CAD build for the part. Positions are in the model's coordinates, mm. Face numbers are marked on the shaded views. A direction names the side the tool comes from. Give positions to 0.01 mm unless a question says otherwise; leave off trailing zeros. Write each loop counter-clockwise with the first axis right and the second up, starting at its lowest first coordinate (ties: lowest second). Pieces come first, ordered by that corner, then holes. Notation, with made-up numbers: (-5.75, 15) - (0.25, 15) arc R5 cw to (0.25, 22) - close; hole circle Ø10 at (70.25, 30.5). An arc over 180 degrees is marked (long way). Answer as a JSON object with one key per item and string values.
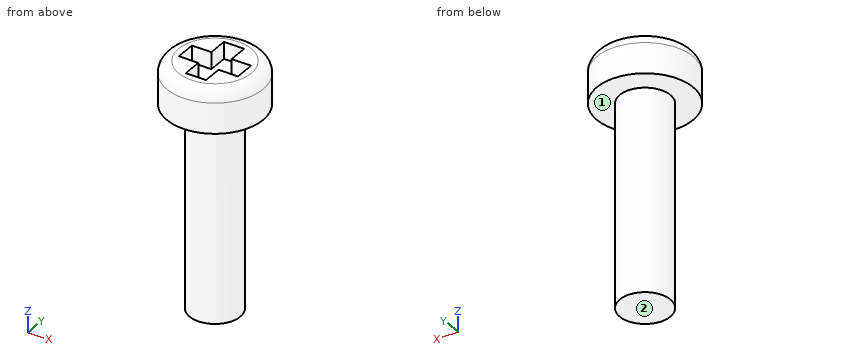
from build123d import *

# Parameters (mm, degrees)
SKETCH_R     = 2.85
PAD_DEPTH    = 2.5
POCKET_DEPTH = 1
FILLET_R     = 0.7
SKETCH002_R  = 1.5
PAD001_DEPTH = 12


with BuildPart() as part:
    # Sketch → Pad (new body)
    with BuildSketch(Plane.XY):
        Circle(SKETCH_R)
    extrude(amount=PAD_DEPTH)

    # Sketch001 (on Face3 of Pad) → Pocket (cut)
    with BuildSketch(Plane.XY.offset(2.5)):
        Polygon((-0.6, 1.75), (0.6, 1.75), (0.6, 0.6), (1.75, 0.6), (1.75, -0.6), (0.6, -0.6), (0.6, -1.75), (-0.6, -1.75), (-0.6, -0.6), (-1.75, -0.6), (-1.75, 0.6), (-0.6, 0.6), align=None)
    extrude(amount=-POCKET_DEPTH, mode=Mode.SUBTRACT)

    # Fillet
    fillet_edges = [part.edges().sort_by_distance(p)[0] for p in [
        (-2.85, 0, 2.5),
    ]]
    fillet(fillet_edges, radius=FILLET_R)

    # Sketch002 (on Face3 of Fillet) → Pad001 (join)
    with BuildSketch(Plane(origin=(0, 0, 0), x_dir=(1, 0, 0), z_dir=(0, 0, -1))):
        Circle(SKETCH002_R)
    extrude(amount=PAD001_DEPTH)


solid = part.part
(1) 3-axis set-ups, long thin cutter, end or side, ignore diameter. For the marked faces 1 and 2: which of +Z, -Z, +X, -X, +Y, -Y reach the whole face in a straight line?
Answer key:
{"face 1": "-Z", "face 2": "-Z, +X, -X, +Y, -Y"}
(2) Flat gauge pins, fed straight in: P1, Ø1.1, axis at y = 1.5, z = 2, coming from the +X side; P2, Ø1, axis at x = 0, y = 0.5, coming from the +Z side; P3, Ø0.5, axis at x = -1, z = 2, coming from the -Y side. Where does each tip first touch, or does it go through?
Answer key:
{"P1": "stops at x = 2.68", "P2": "stops at z = 1.5", "P3": "stops at y = -2.74"}
(3) Saw through at C-C, the plane z = -4.25. Give the cut face in (x, y).
Answer key:
{"outline": "circle Ø3 at (0, 0)"}
(4) Probe L1, parallel to Z at x = 0.8, y = 1.65; L2, parallel to Z at x = 0.3, y = 0.2; L3, parallel to Y at x = -0.1, z = -3.75. List the from-to ranges inside material, lowest first. Write a range as [from, to].
Answer key:
{"L1": "z = [0, 2.5]", "L2": "z = [-12, 1.5]", "L3": "y = [-1.5, 1.5]"}
(5) Saw through at A-A, the plane x = 0. Give the cut face in (y, z).
Answer key:
{"outline": "(-2.85, 0) - (-1.5, 0) - (-1.5, -12) - (1.5, -12) - (1.5, 0) - (2.85, 0) - (2.85, 1.8) arc R0.7 ccw to (2.15, 2.5) - (1.75, 2.5) - (1.75, 1.5) - (-1.75, 1.5) - (-1.75, 2.5) - (-2.15, 2.5) arc R0.7 ccw to (-2.85, 1.8) - close"}
